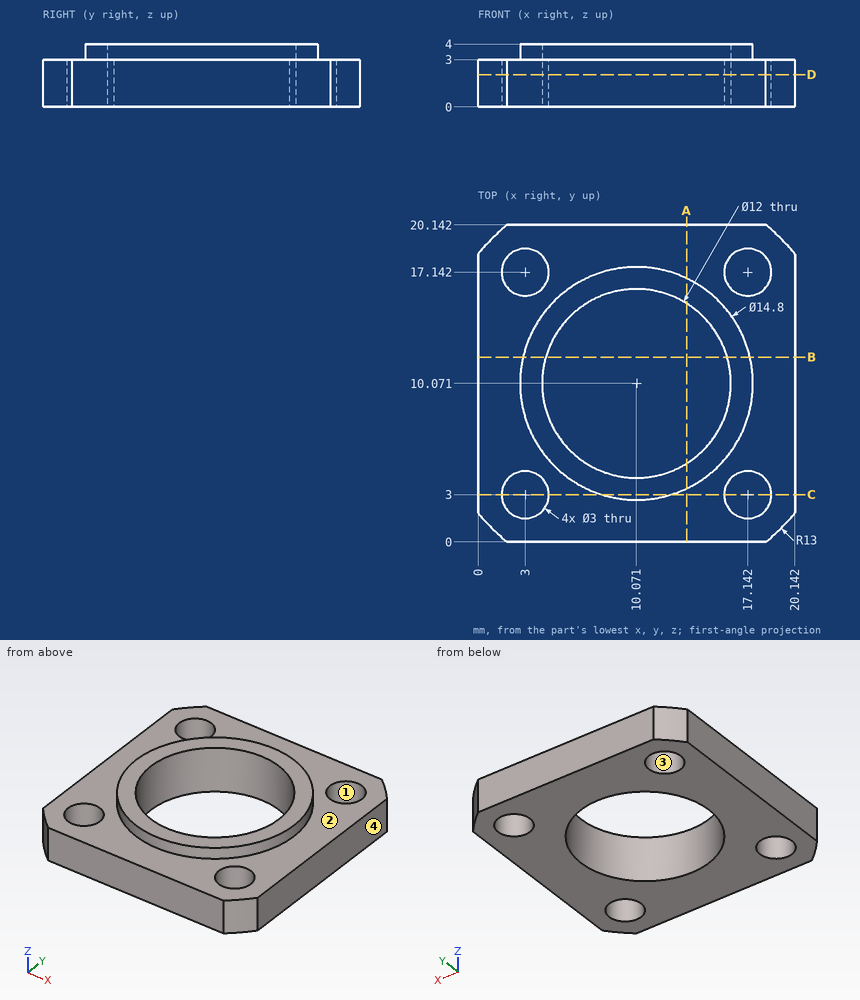
Could you check a few things on this drawing? It's one solid part, dimensions in mm from its lowest x, y, z. Coordinates: 2 decimals unless noted, no trailing zeros. Loops run counter-clockwise (first coordinate to the right, second up) from the corner with the lowest first, then second, coordinate; pieces in that order, holes last. Notation, with made-up numbers: (26, 75.5) - (30, 75.5) arc R26 cw to (30, 107.5) - close; hole circle Ø8 at (43, 37.5). An arc over 180 degrees is marked (long way). Answer as a JSON object with one key per item and string values. Group by question number.
Item 1: If we section it at B-B (y = 11.75): List the corners of the cut face in (x, z) for me.
Item 2: If I drill on L1, parallel to Y at x = 3, z = 1.2; L2, parallel to X at y = 18.5, z = 0.3 (1 decimal); L3, parallel to Y at x = 16.25, z = 2.9, over which ranges is the centre line in solid material (lowest first)? Write a range as from..to.
Item 3: For pin 1 (2 mm diameter, centred on x = 5.5, y = 7.5, fed in from +Z), with a flat end and sliding along its axis, tell me the tip position at first contact or that it passes through.
Item 4: If we section it at A-A (x = 13.25): List the corners of the cut face in (y, z) for me, plus the area to 3 significant figures.
Item 5: If we section it at D-D (z = 2.05): List the corners of the cut face in (x, y) for me, plus the area to 3 significant figures.
Item 6: If we mould it in two halves opening along X, with no side actions, what happens to the marked faces 1, 2, 3 and 4? For each: released by +X, released by -X, zero draft, split by the parting line, or undercut.
Item 7: If we section it at C-C (y = 3): List the corners of the cut face in (x, z) for me, plus the area to 3 significant figures.
Returned:
{
 "1": {"outline": "(0, 0) - (4.31, 0) - (4.31, 4) - (2.86, 4) - (2.86, 3) - (0, 3) - close; (15.83, 0) - (20.14, 0) - (20.14, 3) - (17.28, 3) - (17.28, 4) - (15.83, 4) - close"},
 "2": {"L1": "y = 0..1.5, 4.5..15.64, 18.64..20.14", "L2": "x = 0.2..2.4, 3.6..16.5, 17.8..20", "L3": "y = 0..1.79, 4.21..15.94, 18.35..20.14"},
 "3": {"pin 1": "stops at z = 4"},
 "4": {"outline": "(0, 0) - (4.98, 0) - (4.98, 4) - (3.39, 4) - (3.39, 3) - (0, 3) - close; (15.16, 0) - (20.14, 0) - (20.14, 3) - (16.75, 3) - (16.75, 4) - (15.16, 4) - close", "area": "33.1 mm²"},
 "5": {"outline": "(0, 1.85) arc R13 ccw to (1.85, 0) - (18.29, 0) arc R13 ccw to (20.14, 1.85) - (20.14, 18.29) arc R13 ccw to (18.29, 20.14) - (1.85, 20.14) arc R13 ccw to (0, 18.29) - close; hole circle Ø3 at (3, 3); hole circle Ø3 at (3, 17.14); hole circle Ø12 at (10.07, 10.07); hole circle Ø3 at (17.14, 3); hole circle Ø3 at (17.14, 17.14)", "area": "258 mm²"},
 "6": {"face 1": "undercut", "face 2": "zero draft", "face 3": "undercut", "face 4": "released by +X"},
 "7": {"outline": "(0, 0) - (1.5, 0) - (1.5, 3) - (0, 3) - close; (4.5, 0) - (15.64, 0) - (15.64, 3) - (12.25, 3) - (12.25, 4) - (7.89, 4) - (7.89, 3) - (4.5, 3) - close; (18.64, 0) - (20.14, 0) - (20.14, 3) - (18.64, 3) - close", "area": "46.8 mm²"}
}
